from build123d import *

# Parameters (mm, degrees)
CUT_EXTRUDE1_DEPTH      = 116.003391254
CUT_EXTRUDE1_DEPTH_BACK = 116.003391254
SKETCH4_R               = 6.858
SKETCH5_R               = 6.858
CUT_EXTRUDE2_DEPTH      = 116.003391321
SKETCH5_3_R             = 10.668
CUT_EXTRUDE3_DEPTH      = 116.003391321
SKETCH6_R               = 6.858
CUT_EXTRUDE4_DEPTH      = 25.4


with BuildPart() as part:
    # Sketch3 → Revolve1 (revolve)
    with BuildSketch(Plane.XY, mode=Mode.PRIVATE) as revolve1_sk:
        Polygon((38.1, 101.6), (0, 101.6), (0, 0), (38.1, 0), (38.1, 37.465), (36.83, 37.465), (36.83, 38.735), (38.1, 38.735), align=None)
    revolve(revolve1_sk.sketch.rotate(Axis((0, 101.6, 0), (0, -1, 0)), 180), axis=Axis((0, 101.6, 0), (0, -1, 0)))

    # Sketch4 → Cut-Extrude1 (cut, two sides: drawn at the far end of the back side and taken through both)
    with BuildSketch(Plane.XY.offset(-CUT_EXTRUDE1_DEPTH_BACK)):
        with Locations((0, 18.7325)):
            Circle(SKETCH4_R)
    extrude(amount=CUT_EXTRUDE1_DEPTH + CUT_EXTRUDE1_DEPTH_BACK, mode=Mode.SUBTRACT)

    # Sketch5 → Cut-Extrude2 (cut, through all)
    with BuildSketch(Plane(origin=(0, 0, 0), x_dir=(0, 0, -1), z_dir=(1, 0, 0))):
        with Locations(Location((0, 18.7325, 0), (0, 0, 90))):
            Circle(SKETCH5_R)
    extrude(amount=CUT_EXTRUDE2_DEPTH, mode=Mode.SUBTRACT)

    # Sketch5_3 → Cut-Extrude3 (cut, through all)
    with BuildSketch(Plane(origin=(0, 0, 0), x_dir=(0, 0, -1), z_dir=(1, 0, 0))):
        with Locations(Location((0, 18.7325, 0), (0, 0, 40.005200885))):
            Circle(SKETCH5_3_R)
    extrude(amount=-CUT_EXTRUDE3_DEPTH, mode=Mode.SUBTRACT)

    # Sketch6 → Cut-Extrude4 (cut)
    with BuildSketch(Plane(origin=(0, 101.6, 0), x_dir=(1, 0, 0), z_dir=(0, 1, 0))):
        with Locations(Location((0, 0, 0), (0, 0, 270))):
            Circle(SKETCH6_R)
    extrude(amount=-CUT_EXTRUDE4_DEPTH, mode=Mode.SUBTRACT)


solid = part.part
Check sheet for the modelled part. Datum: model origin and axes. Units: mm. A direction names the side the tool comes from. Coordinates: 2 decimals unless noted, no trailing zeros. Loops run counter-clockwise (first coordinate to the right, second up) from the corner with the lowest first, then second, coordinate; pieces in that order, holes last. Notation, with made-up numbers: (51, 18) -> (85, 18) arc R10 cw to (85, 30) -> close; hole circle Ø11 at (4.5, -18.75). An arc over 180 degrees is marked (long way). Answer in a Markdown table with one row per item.
1. Access from +Z, -Z, +X, -X, +Y, -Y to the whole of each face (thin tool, end or side, straight path). Record for faces 4 (the face through (8.259, 70.608, 37.194)), 5 (the face through (0, 10, 0)), 6 (the face through (0, 76.2, 0)), 7 (the face through (-19.9, 38.735, -31.2)).
Check values:
| item | result |
|---|---|
| face 4 | +Y, -Y |
| face 5 | -X |
| face 6 | +Y |
| face 7 | none |
2. Sectioned sample at D-D, the plane y = 21.5. Record the boundary of the cut face in (x, z), then the cut area to 3 significant figures.
Check values:
| item | result |
|---|---|
| outline | (-36.68, -10.3) arc R38.1 ccw to (-6.27, -37.58) -> (-6.27, -10.3) -> close; (-36.68, 10.3) -> (-6.27, 10.3) -> (-6.27, 37.58) arc R38.1 ccw to start; (6.27, -37.58) arc R38.1 ccw to (37.58, -6.27) -> (6.27, -6.27) -> close; (6.27, 6.27) -> (37.58, 6.27) arc R38.1 ccw to (6.27, 37.58) -> close |
| area | 2,570 mm2 |
3. Sectioned sample at B-B, the plane z = -13.5. Record the boundary of the cut face in (x, y) (1 decimal), then the cut area to 3 significant figures.
Check values:
| item | result |
|---|---|
| outline | (-35.6, 0) -> (35.6, 0) -> (35.6, 37.5) -> (34.3, 37.5) -> (34.3, 38.7) -> (35.6, 38.7) -> (35.6, 101.6) -> (-35.6, 101.6) -> (-35.6, 38.7) -> (-34.3, 38.7) -> (-34.3, 37.5) -> (-35.6, 37.5) -> close; hole circle Ø13.7 at (0, 18.7) |
| area | 7,090 mm2 |
4. Release check for a two-part mould opening along Y. For faces 1 (the face through (-1, 0, -1)), 2 (the face through (-6.695, 89.078, -1.487)), 3 (the face through (6.54, 20.79, 23.02)) record: released by +Y, released by -Y, zero draft, split by the parting line, or undercut.
Check values:
| item | result |
|---|---|
| face 1 | released by -Y |
| face 2 | zero draft |
| face 3 | undercut |
5. Material ranges on line 1 along Y through (x, z) = (0, -18); line 2 along X through (y, z) = (25, 13); line 3 along X through (y, z) = (19, 24.5), recorded low to high. Write a range as [from, to].
Check values:
| item | result |
|---|---|
| line 1 | y = [0, 11.87], [25.59, 101.6] |
| line 2 | x = [-35.81, -2.78], [2.78, 35.81] |
| line 3 | x = [-29.18, -6.85], [6.85, 29.18] |
6. Sectioned sample at A-A, the plane x = -2. Record the boundary of the cut face in (y, z) (1 decimal), then the cut area to 3 significant figures.
Check values:
| item | result |
|---|---|
| outline | (0, -38) -> (12.2, -38) -> (12.2, -8.4) arc R10.7 cw to (12.2, 8.4) -> (12.2, 38) -> (0, 38) -> close; (25.3, -38) -> (37.5, -38) -> (37.5, -36.8) -> (38.7, -36.8) -> (38.7, -38) -> (101.6, -38) -> (101.6, -6.6) -> (76.2, -6.6) -> (76.2, 6.6) -> (101.6, 6.6) -> (101.6, 38) -> (38.7, 38) -> (38.7, 36.8) -> (37.5, 36.8) -> (37.5, 38) -> (25.3, 38) -> (25.3, 8.4) arc R10.7 cw to (25.3, -8.4) -> close |
| area | 6,300 mm2 |
7. Sectioned sample at C-C, the plane z = 2.5. Record the boundary of the cut face in (x, y) (1 decimal), then the cut area to 3 significant figures.
Check values:
| item | result |
|---|---|
| outline | (-38, 0) -> (38, 0) -> (38, 12.3) -> (2.5, 12.3) arc R6.9 cw to (0, 11.9) -> (0, 8.4) -> (-38, 8.4) -> close; (-38, 29.1) -> (0, 29.1) -> (0, 25.6) arc R6.9 cw to (2.5, 25.1) -> (38, 25.1) -> (38, 37.5) -> (36.7, 37.5) -> (36.7, 38.7) -> (38, 38.7) -> (38, 101.6) -> (6.4, 101.6) -> (6.4, 76.2) -> (-6.4, 76.2) -> (-6.4, 101.6) -> (-38, 101.6) -> (-38, 38.7) -> (-36.7, 38.7) -> (-36.7, 37.5) -> (-38, 37.5) -> close |
| area | 6,120 mm2 |
8. Go/stop test with flat-tipped pins: pin 1 (1.1 mm diameter, centred on y = 27, z = -2.5, fed in from -X); pin 2 (8 mm diameter, centred on x = -20, y = 88.5, fed in from +Z); pin 3 (3 mm diameter, centred on y = 55.5, z = -2, fed in from -X); pin 4 (8 mm diameter, centred on x = 0, y = 18.73, fed in from -Z). Record where each tip stops, or that it passes through.
Check values:
| item | result |
|---|---|
| pin 1 | stops at x = 0 |
| pin 2 | stops at z = 34.58 |
| pin 3 | stops at x = -38.1 |
| pin 4 | passes through |
